from build123d import *

# Parameters (mm, degrees)
SKETCH161_R  = 1.8
PAD126_DEPTH = 3.35
SKETCH158_R  = 1.8
PAD123_DEPTH = 4
SKETCH159_R  = 1.8
SKETCH159_W  = 2.5
SKETCH159_H  = 13
PAD124_DEPTH = 4
SKETCH156_R  = 1.7
PAD121_DEPTH = 60


with BuildPart() as motorcageringcutout:
    # Sketch161 → Pad126 (new body)
    with BuildSketch(Plane.XZ.offset(-53)):
        with BuildLine():
            Line((-16.85, 24), (-23.5, 12.481862))
            Line((-23.5, 12.481862), (-23.5, 7.75))
            Line((-23.5, 7.75), (-26.2, 7.75))
            Line((-26.2, 7.75), (-28.95, 5))
            Line((-28.95, 5), (-26.2, 2.25))
            Line((-26.2, 2.25), (-23.5, 2.25))
            Line((-23.5, 2.25), (-23.5, -2.25))
            Line((-23.5, -2.25), (-26.2, -2.25))
            Line((-26.2, -2.25), (-28.95, -5))
            Line((-28.95, -5), (-26.2, -7.75))
            Line((-26.2, -7.75), (-23.5, -7.75))
            Line((-23.5, -7.75), (-23.5, -12.473721))
            Line((-23.5, -12.473721), (-18, -22))
            Line((-18, -22), (0, -22))
            Line((0, -18.35), (0, -22))
            ThreePointArc((0, 18.35), (-18.35, 0), (0, -18.35))
            Line((0, 24), (0, 18.35))
            Line((-16.85, 24), (0, 24))
        make_face()
        with Locations((-15, 21)):
            Circle(SKETCH161_R, mode=Mode.SUBTRACT)
        with Locations((-15, -17)):
            Circle(SKETCH161_R, mode=Mode.SUBTRACT)
    extrude(amount=-PAD126_DEPTH)


with BuildPart() as endcap:
    # Sketch158 → Pad123 (new body)
    with BuildSketch(Plane.XZ.offset(-30)):
        Polygon((-29.490381, 15), (-39.5, 9.220944), (-39.5, -9.220944), (-29.490381, -15), (-24, -11.830127), (-24, 11.830127), align=None)
        with Locations((-29, 10)):
            Circle(SKETCH158_R, mode=Mode.SUBTRACT)
        with Locations((-29, -10)):
            Circle(SKETCH158_R, mode=Mode.SUBTRACT)
        with Locations((-36, 0)):
            Circle(SKETCH158_R, mode=Mode.SUBTRACT)
    extrude(amount=-PAD123_DEPTH)


with BuildPart() as pad124:
    # Sketch159 → Pad124 (new body)
    with BuildSketch(Plane.XZ.offset(-90)):
        Polygon((-29.490381, 15), (-39.5, 9.220944), (-39.5, -9.220944), (-29.490381, -15), (-24, -11.830127), (-24, 11.830127), align=None)
        with Locations((-29, 10)):
            Circle(SKETCH159_R, mode=Mode.SUBTRACT)
        with Locations((-29, -10)):
            Circle(SKETCH159_R, mode=Mode.SUBTRACT)
        with Locations((-36, 0)):
            Circle(SKETCH159_R, mode=Mode.SUBTRACT)
        with Locations((-30.25, 0)):
            Rectangle(SKETCH159_W, SKETCH159_H, mode=Mode.SUBTRACT)
    extrude(amount=PAD124_DEPTH)


with BuildPart() as sidewall:
    # Sketch156 → Pad121 (new body)
    with BuildSketch(Plane.XZ.offset(-30)):
        Polygon((-29.490381, 15), (-34.5, 12.107695), (-31.5, 4), (-31.5, 3.75), (-29.5, 6.25), (-29, 6.25), (-29, -6.25), (-29.5, -6.25), (-31.5, -3.75), (-31.5, -4), (-34.5, -12.107695), (-29.490381, -15), (-24, -11.830127), (-24, 11.830127), align=None)
        with Locations((-29, 10)):
            Circle(SKETCH156_R, mode=Mode.SUBTRACT)
        with Locations((-29, -10)):
            Circle(SKETCH156_R, mode=Mode.SUBTRACT)
    extrude(amount=-PAD121_DEPTH)

    # Fusion004020009: union EndCap, Pad124
    add(endcap.part)
    add(pad124.part)

    # Cut007019014: cut MotorCageRingCutout
    add(motorcageringcutout.part, mode=Mode.SUBTRACT)


with BuildPart() as part_mirroring018:
    # Part__Mirroring018: instance of SideWall
    add(sidewall.part.mirror(Plane(origin=(0, 0, 0), x_dir=(0, -1, 0), z_dir=(1, 0, 0))))


solid = part_mirroring018.part
Input: part model. Units: mm. Frame: model coordinates. A direction names the side the tool comes from. Coordinates: 2 decimals unless noted, no trailing zeros. Order: outer loops, then holes, each group sorted by start corner. A loop starts at its lowest first (then second) coordinate and runs counter-clockwise, first axis right, second up.
1. Access query for faces 1 (the cylindrical face through (34.283, 31.972, 0.541)), 2 (the flat face through (30.5, 61.6, -5)), 3 (the flat face through (34, 86, 0)), 4 (the flat face through (25, 55, -7.75)). Directions: +Z, -Z, +X, -X, +Y, -Y. A direction counts if a zero-diameter tool reaches every point of the face in a straight line with its end or side. Return the directions, or none.
Checked values:
face 1: +Y, -Y
face 2: +Y
face 3: +X
face 4: -X
2. Contact query for flat-ended pins moving along their axis: P1, Ø10, axis at y = 75, z = 0, coming from the +X side; P2, Ø1.1, axis at x = 25, y = 55, coming from the +Z side (3 decimals); P3, Ø2, axis at y = 62, z = 6.5, coming from the +X side. Output: stop coordinate, or through.
Checked values:
P1: stops at x = 31.87
P2: stops at z = 12.725
P3: stops at x = 32.8
3. Ray query, line 1 along Y through (x, z) = (34, 0); line 2 along Z through (x, y) = (28, 61.5); line 3 along Z through (x, y) = (28.5, 37). Return the intervals inside material, ascending.
Checked values:
line 1: y = 30 to 34, 86 to 90
line 2: z = -14.14 to -11.37, -8.63 to 8.63, 11.37 to 14.14
line 3: z = -14.43 to -11.62, -8.38 to 8.38, 11.62 to 14.43
4. Cut plane C-C, the plane y = 42.5. Return loops of the section in (x, z).
Checked values:
outline: (24, -11.83) - (29.49, -15) - (34.5, -12.11) - (31.5, -4) - (31.5, -3.75) - (29.5, -6.25) - (29, -6.25) - (29, 6.25) - (29.5, 6.25) - (31.5, 3.75) - (31.5, 4) - (34.5, 12.11) - (29.49, 15) - (24, 11.83) - close; hole circle Ø3.4 at (29, -10); hole circle Ø3.4 at (29, 10)
5. Draft query along Z for faces 5 (the flat face through (26.707, 59.58, 13.393)), 6 (the flat face through (32, 90, 0)), 7 (the flat face through (26, 53, 5)), 8 (the cylindrical face through (27.43, 59.58, -10.65)). Return one class per face: +Z half, -Z half, draft (parallel to the pull), parting line (faces both ways), or undercut.
Checked values:
face 5: +Z half
face 6: draft
face 7: undercut
face 8: undercut
6. Cut plane A-A, the plane z = 0. Return loops of the section in (x, y), plus the area to 3 significant figures.
Checked values:
outline: (24, 30) - (34.2, 30) - (34.2, 34) - (29, 34) - (29, 90) - (24, 90) - close; (31.5, 86) - (34.2, 86) - (34.2, 90) - (31.5, 90) - close; (37.8, 30) - (39.5, 30) - (39.5, 34) - (37.8, 34) - close; (37.8, 86) - (39.5, 86) - (39.5, 90) - (37.8, 90) - close
area: 345 mm2
7. Cut plane B-B, the plane x = 36.75. Return loops of the section in (y, z), plus the area to 3 significant figures.
Checked values:
outline: (30, -10.81) - (34, -10.81) - (34, -1.64) - (30, -1.64) - close; (30, 1.64) - (34, 1.64) - (34, 10.81) - (30, 10.81) - close; (86, -10.81) - (90, -10.81) - (90, -1.64) - (86, -1.64) - close; (86, 1.64) - (90, 1.64) - (90, 10.81) - (86, 10.81) - close
area: 147 mm2
